Autodesk Fusion 360 part; units mm, degrees
sketch "Sketch1" plane through (0, 0, 0) normal (0, 0, 1) x (1, 0, 0)
  line L0 (-8.0882, 5) -> (41.9118, 5)
  line L1 (41.9118, 5) -> (41.9118, 205)
  line L2 (41.9118, 205) -> (-8.0882, 205)
  line L3 (-8.0882, 205) -> (-8.0882, 5)
  line L4 (-8.0882, 205) -> (-3.8456, 200.7574)
  line L5 (-8.0882, 205) -> (6, 205) construction
  line L6 (-8.0882, 5) -> (-3.8456, 9.2426)
  line L7 (-8.0882, 5) -> (6, 5) construction
  line L8 (16.9118, 205) -> (16.9118, 5)
  circle A0 centre (-3.8456, 200.7574) radius 1.75
  circle A1 centre (-3.8456, 9.2426) radius 1.75
  circle A2 centre (37.6691, 200.7574) radius 1.75
  circle A3 centre (37.6691, 9.2426) radius 1.75
  dimension "d1" = 200
  dimension "d2" = 50
  dimension "d3" = 6
  dimension "d4" = 45
  dimension "d5" = 45
  dimension "d6" = 6
  dimension "d7" = 3.5
  dimension "d8" = 3.5
extrude "Extrude1" add sketch "Sketch1" along normal blind 3
sketch "Sketch2" plane through (0, 0, 3) normal (0, 0, 1) x (1, 0, 0)
  circle A0 centre (-3.8456, 200.7574) radius 1.75
  circle A1 centre (37.6691, 9.2426) radius 1.75
  circle A2 centre (-3.8456, 9.2426) radius 1.75
  circle A3 centre (37.6691, 200.7574) radius 1.75
  line L0 (-8.0882, 205) -> (-8.0882, 5)
  line L1 (-8.0882, 5) -> (41.9118, 5)
  line L2 (41.9118, 5) -> (41.9118, 205)
  line L3 (41.9118, 205) -> (-8.0882, 205)
  line L4 (41.9118, 5) -> (29.4118, 5)
  line L5 (29.4118, 205) -> (41.9118, 205)
  line L6 (41.9118, 205) -> (41.9118, 5)
  line L7 (-8.0882, 5) -> (4.4118, 5)
  line L8 (4.4118, 205) -> (-8.0882, 205)
  line L9 (-8.0882, 205) -> (-8.0882, 5)
  line L10 (-8.0882, 205) -> (-8.0882, 180)
  line L11 (-8.0882, 5) -> (-8.0882, 30)
  circle A4 centre (4.4118, 180) radius 4.75
  circle A5 centre (4.4118, 152.5) radius 4.75
  circle A6 centre (4.4118, 125) radius 4.75
  circle A7 centre (4.4118, 97.5) radius 4.75
  circle A8 centre (29.4118, 152.5) radius 4.75
  circle A9 centre (29.4118, 125) radius 4.75
  circle A10 centre (29.4118, 180) radius 4.75
  circle A11 centre (29.4118, 97.5) radius 4.75
  circle A12 centre (16.9118, 61.25) radius 7.75
  circle A13 centre (5.8118, 61.25) radius 1.6
  circle A14 centre (28.0118, 61.25) radius 1.6
  line L12 (16.9118, 50.625) -> (-8.0882, 50.625)
  line L13 (-8.0882, 50.625) -> (41.9118, 50.625)
  circle A15 centre (16.9118, 40) radius 7.75
  circle A16 centre (28.0118, 40) radius 1.6
  circle A17 centre (5.8118, 40) radius 1.6
  point P0 (28.0118, 40)
  point P1 (5.8118, 40)
  dimension "d11" = 12.5
  dimension "d12" = 200
  dimension "d13" = 12.5
  dimension "d14" = 200
  dimension "d15" = 9.5
  dimension "d17" = 27.5
  dimension "d18" = 9.5
  dimension "d19" = 27.5
  dimension "d20" = 9.5
  dimension "d21" = 27.5
  dimension "d22" = 9.5
  dimension "d23" = 92.5
  dimension "d25" = 15.5
  dimension "d26" = 11.1
  dimension "d27" = 3.2
extrude "Extrude2" cut sketch "Sketch2" against normal blind 3 contours A4 | A5 | A6 | A7 | A8 | A9 | A10 | A11 | A12 | A13 | A14
sketch "Sketch3" plane through (0, 0, 0) normal (0, 0, -1) x (-1, 0, 0)
  circle A0 centre (-4.4118, 152.5) radius 4.75
  circle A1 centre (-29.4118, 97.5) radius 4.75
  circle A2 centre (-16.9118, 61.25) radius 7.75
  circle A3 centre (-4.4118, 97.5) radius 4.75
  circle A4 centre (-29.4118, 152.5) radius 4.75
  circle A5 centre (-4.4118, 180) radius 4.75
  circle A6 centre (-29.4118, 125) radius 4.75
  circle A7 centre (-28.0118, 61.25) radius 1.6
  circle A8 centre (-5.8118, 61.25) radius 1.6
  circle A9 centre (-4.4118, 125) radius 4.75
  circle A10 centre (-29.4118, 180) radius 4.75
  circle A11 centre (3.8456, 200.7574) radius 1.75
  circle A12 centre (-37.6691, 9.2426) radius 1.75
  circle A13 centre (3.8456, 9.2426) radius 1.75
  circle A14 centre (-37.6691, 200.7574) radius 1.75
  line L0 (8.0882, 5) -> (8.0882, 205)
  line L1 (8.0882, 205) -> (-41.9118, 205)
  line L2 (-41.9118, 205) -> (-41.9118, 5)
  line L3 (-41.9118, 5) -> (8.0882, 5)
  line L4 (-41.9118, 205) -> (-38.9118, 205)
  line L5 (-38.9118, 205) -> (-38.9118, 190)
  line L6 (-38.9118, 190) -> (-41.9118, 190)
  line L7 (-41.9118, 190) -> (-41.9118, 205)
  line L8 (-16.9118, 205) -> (-16.9118, 5)
  line L9 (8.0882, 205) -> (5.0882, 205)
  line L10 (5.0882, 205) -> (5.0882, 190)
  line L11 (5.0882, 190) -> (8.0882, 190)
  line L12 (8.0882, 190) -> (8.0882, 205)
  line L13 (-41.9118, 5) -> (-38.9118, 5)
  line L14 (-38.9118, 5) -> (-38.9118, 20)
  line L15 (-38.9118, 20) -> (-41.9118, 20)
  line L16 (-41.9118, 20) -> (-41.9118, 5)
  line L17 (8.0882, 5) -> (5.0882, 5)
  line L18 (5.0882, 5) -> (5.0882, 20)
  line L19 (5.0882, 20) -> (8.0882, 20)
  line L20 (8.0882, 20) -> (8.0882, 5)
  line L21 (-41.9118, 190) -> (-38.9118, 190)
  line L22 (-38.9118, 190) -> (-38.9118, 20)
  line L23 (-38.9118, 20) -> (-41.9118, 20)
  line L24 (-41.9118, 20) -> (-41.9118, 190)
  line L25 (5.0882, 190) -> (8.0882, 190)
  line L26 (8.0882, 190) -> (8.0882, 20)
  line L27 (8.0882, 20) -> (5.0882, 20)
  line L28 (5.0882, 20) -> (5.0882, 190)
  dimension "d30" = 3
  dimension "d31" = 15
  dimension "d32" = 3
  dimension "d33" = 15
  dimension "d34" = 3
  dimension "d35" = 15
  dimension "d36" = 3
  dimension "d37" = 15
extrude "Extrude3" add sketch "Sketch3" along normal blind 5 contours L0 L11 L19 L25 L26 L27 L28 | L2 L6 L15 L21 L22 L23 L24
sketch "Sketch4" plane through (0, 0, 0) normal (0, 0, -1) x (-1, 0, 0)
  circle A0 centre (-37.6691, 200.7574) radius 1.75
  circle A1 centre (3.8456, 9.2426) radius 1.75
  circle A2 centre (-37.6691, 9.2426) radius 1.75
  circle A3 centre (3.8456, 200.7574) radius 1.75
  circle A4 centre (-29.4118, 180) radius 4.75
  circle A5 centre (-4.4118, 125) radius 4.75
  circle A6 centre (-5.8118, 61.25) radius 1.6
  circle A7 centre (-28.0118, 61.25) radius 1.6
  circle A8 centre (-29.4118, 125) radius 4.75
  circle A9 centre (-4.4118, 180) radius 4.75
  circle A10 centre (-29.4118, 152.5) radius 4.75
  circle A11 centre (-4.4118, 97.5) radius 4.75
  circle A12 centre (-16.9118, 61.25) radius 7.75
  circle A13 centre (-29.4118, 97.5) radius 4.75
  circle A14 centre (-4.4118, 152.5) radius 4.75
  line L0 (-41.9118, 190) -> (-38.9118, 190)
  line L1 (-38.9118, 190) -> (-38.9118, 20)
  line L2 (-38.9118, 20) -> (-41.9118, 20)
  line L3 (-41.9118, 20) -> (-41.9118, 5)
  line L4 (-41.9118, 5) -> (8.0882, 5)
  line L5 (8.0882, 5) -> (8.0882, 20)
  line L6 (8.0882, 20) -> (5.0882, 20)
  line L7 (5.0882, 20) -> (5.0882, 190)
  line L8 (5.0882, 190) -> (8.0882, 190)
  line L9 (8.0882, 190) -> (8.0882, 205)
  line L10 (8.0882, 205) -> (-41.9118, 205)
  line L11 (-41.9118, 205) -> (-41.9118, 190)
  line L12 (-38.9118, 20) -> (-38.9118, 30)
  line L13 (-38.9118, 30) -> (-35.9118, 30)
  line L14 (-35.9118, 30) -> (-35.9118, 40)
  line L15 (-35.9118, 40) -> (-38.9118, 40)
  line L16 (-38.9118, 40) -> (-38.9118, 30)
  line L17 (-38.9118, 40) -> (-38.9118, 87)
  line L18 (-38.9118, 87) -> (-35.9118, 87)
  line L19 (-35.9118, 87) -> (-35.9118, 97)
  line L20 (-35.9118, 97) -> (-38.9118, 97)
  line L21 (-38.9118, 97) -> (-38.9118, 87)
  dimension "d40" = 3
  dimension "d41" = 10
  dimension "d42" = 47
  dimension "d43" = 3
  dimension "d44" = 10
extrude "Extrude4" add sketch "Sketch4" along normal blind 20 contours L1 L18 L19 L20 L21 | L1 L13 L14 L15 L16
fillet "Fillet1" radius 3.5 4 edges at (37.4118, 87, -20) (37.4118, 97, -20) (37.4118, 30, -20) (37.4118, 40, -20)
chamfer "Chamfer1" distance 5 angle 45 2 edges at (40.4118, 20, -5) (-6.5882, 20, -5)
chamfer "Chamfer2" distance 5 angle 45 2 edges at (-6.5882, 190, -5) (40.4118, 190, -5)
sketch "Sketch5" plane through (35.9118, 0, 0) normal (-1, 0, 0) x (0, 0, 1)
  arc A0 (-16.5, 97) -> (-20, 93.5) centre (-16.5, 93.5) ccw
  line L0 (-20, 93.5) -> (-20, 90.5)
  arc A1 (-20, 90.5) -> (-16.5, 87) centre (-16.5, 90.5) ccw
  line L1 (-16.5, 87) -> (0, 87)
  line L2 (0, 87) -> (0, 97)
  line L3 (0, 97) -> (-16.5, 97)
  line L4 (-20, 92) -> (-16, 92)
  circle A2 centre (-16, 92) radius 1.75
  line L5 (-20, 35) -> (-16, 35)
  circle A3 centre (-16, 35) radius 1.75
  dimension "d50" = 4
  dimension "d51" = 3.5
  dimension "d52" = 3.5
extrude "Extrude5" cut sketch "Sketch5" against normal blind 5 contours A2 | A3
extrude "Extrude6" cut sketch "Sketch2" against normal blind 3 contours A15
extrude "Extrude7" cut sketch "Sketch2" against normal blind 3 contours A16 | A17
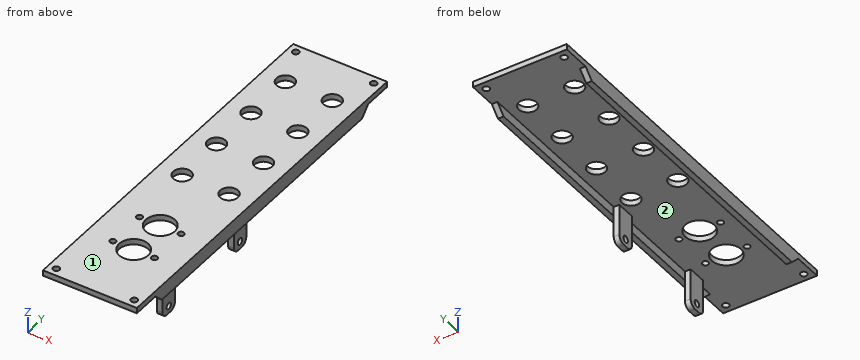
The model under review builds one solid part; all positions refer to its coordinate system, in mm. Face numbers are marked on the shaded views. Coordinates: 2 decimals unless noted, no trailing zeros. Order: outer loops, then holes, each group sorted by start corner. A loop starts at its lowest first (then second) coordinate and runs counter-clockwise, first axis right, second up. Notation, with made-up numbers: (79, -25.75) -> (109, -25.75) arc R37 cw to (109, 13.25) -> close; hole circle Ø1 at (-1.75, 65.25). An arc over 180 degrees is marked (long way). Answer in a Markdown table with one row per item. Add a question column.
Item 1: We need section C-C on x = 14.5. Write out the cut boundary in (y, z), plus the area to 3 significant figures.
Item 2: Clearance check with flat-ended pins moving along their axes: pin 1 (2.5 mm diameter, centred on x = 40, y = 119, fed in from -Z); pin 2 (4.5 mm diameter, centred on y = 35, z = -16, fed in from +X); pin 3 (3.5 mm diameter, centred on x = 37.5, z = -9, fed in from +Y). State where each tip first meets the part, or that it passes through.
Item 3: To check wall thickness, follow probe 1 along X at (y, z) = (145, -1.5); probe 2 along Z at (x, y) = (38, 92); probe 3 along X at (y, z) = (32.5, -4.5). State the ranges of each line that lie inside material, in increasing order.
Item 4: We need section D-D on y = 160. Write out the cut boundary in (x, z).
Item 5: We need section A-A on y = 125. Write out the cut boundary in (x, z), plus the area to 3 significant figures.
Item 6: We need section B-B on y = 67. Write out the cut boundary in (x, z), plus the area to 3 significant figures.
Item 7: Mouldability with a two-part tool opening along X and no side actions: class the marked faces 1 and 2 as +X half, -X half, draft (parallel to the pull), parting line (faces both ways), or undercut.
Final values:
| question | item | result |
|---|---|---|
| 1 | outline | (5, 0) -> (32.63, 0) -> (32.63, 3) -> (5, 3) -> close; (47.37, 0) -> (53.88, 0) -> (53.88, 3) -> (47.37, 3) -> close; (68.62, 0) -> (205, 0) -> (205, 3) -> (68.62, 3) -> close |
| 1 | area | 512 mm2 |
| 2 | pin 1 | stops at z = -5 |
| 2 | pin 2 | stops at x = 38.91 |
| 2 | pin 3 | stops at y = 97 |
| 3 | probe 1 | x = -8.09 to -5.09, 38.91 to 41.91 |
| 3 | probe 2 | z = -20 to -17.75, -14.25 to 3 |
| 3 | probe 3 | x = -8.09 to -5.09, 35.91 to 41.91 |
| 4 | outline | (-8.09, -5) -> (-5.09, -5) -> (-5.09, 0) -> (38.91, 0) -> (38.91, -5) -> (41.91, -5) -> (41.91, 3) -> (-8.09, 3) -> close |
| 5 | outline | (-8.09, -5) -> (-5.09, -5) -> (-5.09, 0) -> (-0.34, 0) -> (-0.34, 3) -> (-8.09, 3) -> close; (9.16, 0) -> (24.66, 0) -> (24.66, 3) -> (9.16, 3) -> close; (34.16, 0) -> (38.91, 0) -> (38.91, -5) -> (41.91, -5) -> (41.91, 3) -> (34.16, 3) -> close |
| 5 | area | 123 mm2 |
| 6 | outline | (-8.09, -5) -> (-5.09, -5) -> (-5.09, 0) -> (11.72, 0) -> (11.72, 3) -> (-8.09, 3) -> close; (22.11, 0) -> (38.91, 0) -> (38.91, -5) -> (41.91, -5) -> (41.91, 3) -> (22.11, 3) -> close |
| 6 | area | 149 mm2 |
| 7 | face 1 | draft |
| 7 | face 2 | undercut |
